Part model, mm, in its own coordinate system. A direction names the side the tool comes from. Give positions to 0.01 mm unless a question says otherwise; leave off trailing zeros. Loops run counter-clockwise (first coordinate to the right, second up) from the corner with the lowest first, then second, coordinate; pieces in that order, holes last. Notation, with made-up numbers: (67.5, -36) -> (75.5, -36) arc R11 ccw to (75.5, -26) -> close; hole circle Ø4 at (5.5, -23.75). An arc over 180 degrees is marked (long way). One line per question, with ' | ' between items.
Autodesk Inventor part; units mm, degrees
ref_plane "YZ Plane" through (0, 0, 0) normal (1, 0, 0) x (0, 1, 0)
ref_plane "XZ Plane" through (0, 0, 0) normal (0, 1, 0) x (-1, 0, 0)
ref_plane "XY Plane" through (0, 0, 0) normal (0, 0, 1) x (1, 0, 0)
sketch "Esquisse1" plane through (0, 0, 0) normal (0, 0, 1) x (1, 0, 0)
  line L0 (0, 0) -> (45, 0)
  line L1 (45, 0) -> (45, 20)
  line L2 (45, 20) -> (0, 20)
  line L3 (0, 20) -> (0, 0)
  dimension "d0" = 45
  dimension "d1" = 20
extrude "Extrusion1" add sketch "Esquisse1" along normal blind 3
sketch "Esquisse2" plane through (0, 0, 3) normal (0, 0, 1) x (1, 0, 0)
  line L0 (45, 0) -> (45, 20)
  line L1 (0, 0) -> (45, 0)
  circle A0 centre (11.5, 10) radius 8
  circle A1 centre (33.5, 10) radius 8
  dimension "d4" = 22
  dimension "d5" = 11.5
  dimension "d6" = 10
  dimension "d7" = 10
  dimension "d8" = 16
  dimension "d9" = 16
extrude "Extrusion2" add sketch "Esquisse2" along normal blind 8
sketch "Esquisse3" plane through (11.5, 10, 11) normal (0, 0, 1) x (1, 0, 0)
  circle A0 centre (0, 0) radius 6.5
  circle A1 centre (22, 0) radius 8
  circle A2 centre (22, 0) radius 6.5
  circle A3 centre (0, 0) radius 7.9442
  circle A4 centre (22, 0) radius 8
  point P0 (-11.5, -10)
  dimension "d12" = 13
  dimension "d13" = 13
extrude "Extrusion3" cut sketch "Esquisse3" against normal blind 2 contours A0 | A2
sketch "Esquisse4" plane through (0, 0, 0) normal (0, -1, 0) x (1, 0, 0)
  line L0 (45, 0) -> (45, 3)
  circle A0 centre (19.5, 1.5) radius 0.75
  circle A1 centre (21.5, 1.5) radius 0.75
  circle A2 centre (23.5, 1.5) radius 0.75
  circle A3 centre (25.5, 1.5) radius 0.75
  line L1 (0, 3) -> (45, 3)
  point P0 (0, 0)
  dimension "d17" = 2
  dimension "d18" = 2
  dimension "d19" = 2
  dimension "d22" = 1.5
  dimension "d23" = 1.5
  dimension "d24" = 1.5
  dimension "d25" = 1.5
  dimension "d26" = 19.5
  dimension "d29" = 1.5
  dimension "d30" = 3
extrude "Extrusion4" add sketch "Esquisse4" along normal blind 7
properties part number "US HC-SR04"
1) Saw through at B-B (z = 6.5). Give the cut face in (x, y).
Found:
outline: circle Ø16 at (11.5, 10); circle Ø16 at (33.5, 10)
2) Saw through at C-C (y = 10). Give the cut face in (x, z), and give its area (3 significant figures).
Found:
outline: (0, 0) -> (45, 0) -> (45, 3) -> (41.5, 3) -> (41.5, 11) -> (40, 11) -> (40, 9) -> (27, 9) -> (27, 11) -> (25.5, 11) -> (25.5, 3) -> (19.5, 3) -> (19.5, 11) -> (18, 11) -> (18, 9) -> (5, 9) -> (5, 11) -> (3.5, 11) -> (3.5, 3) -> (0, 3) -> close | area: 339 mm2
3) Drill centre lines: line 1 (Y direction, x = 33.5, z = 10); line 2 (Z direction, x = 4, y = 4.75); line 3 (Z direction, x = 16, y = 11.5). Where is each one in solid material? Low to high.
Found:
line 1: 2 to 3.5, 16.5 to 18 | line 2: 0 to 3 | line 3: 0 to 9
4) Saw through at A-A (x = 33.5). Give the cut face in (y, z), and give its area (3 significant figures).
Found:
outline: (0, 0) -> (20, 0) -> (20, 3) -> (18, 3) -> (18, 11) -> (16.5, 11) -> (16.5, 9) -> (3.5, 9) -> (3.5, 11) -> (2, 11) -> (2, 3) -> (0, 3) -> close | area: 162 mm2
5) Pull direction X, two halves, no side cores. Call faces 1 (the cylindrical face through (32.654, 16.445, 10.014)), 2 (the flat face through (23, 20, 1)), 3 (the flat face through (45, 10, 1)): pulls with the +X half, pulls with the -X half, needs draft (parallel to the pull), parting line crosses it, or undercut.
Found:
face 1: undercut | face 2: needs draft | face 3: pulls with the +X half
6) Pin check, flat tips, straight feed: P1, Ø10.5, axis at x = 11.5, y = 10, coming from the +Z side; P2, Ø14.5, axis at x = 33.5, y = 10, coming from the +Z side; P3, Ø4, axis at x = 9.5, z = 5.5, coming from the -Y side; P4, Ø1.5, axis at x = 26, y = -2, coming from the +Z side. Stop position of each tip, or through.
Found:
P1: z = 9 | P2: z = 11 | P3: y = 2 | P4: z = 2.25
7) Tool access for faces 4 (the cylindrical face through (20.75, -3.45, 1.47)), 5 (the cylindrical face through (9.77, 17.81, 6.94)), 6 (the flat face through (11, 17, 11)): list every direction of +Z, -Z, +X, -X, +Y, -Y with a clear straight run to the whole face (end or side of a thin tool).
Found:
face 4: -Y | face 5: +Z | face 6: +Z, +X, -X, +Y, -Y
8) Saw through at D-D (z = 10). Give the cut face in (x, y), and give its area (3 significant figures).
Found:
outline: circle Ø16 at (11.5, 10); circle Ø16 at (33.5, 10); hole circle Ø13 at (11.5, 10); hole circle Ø13 at (33.5, 10) | area: 137 mm2
